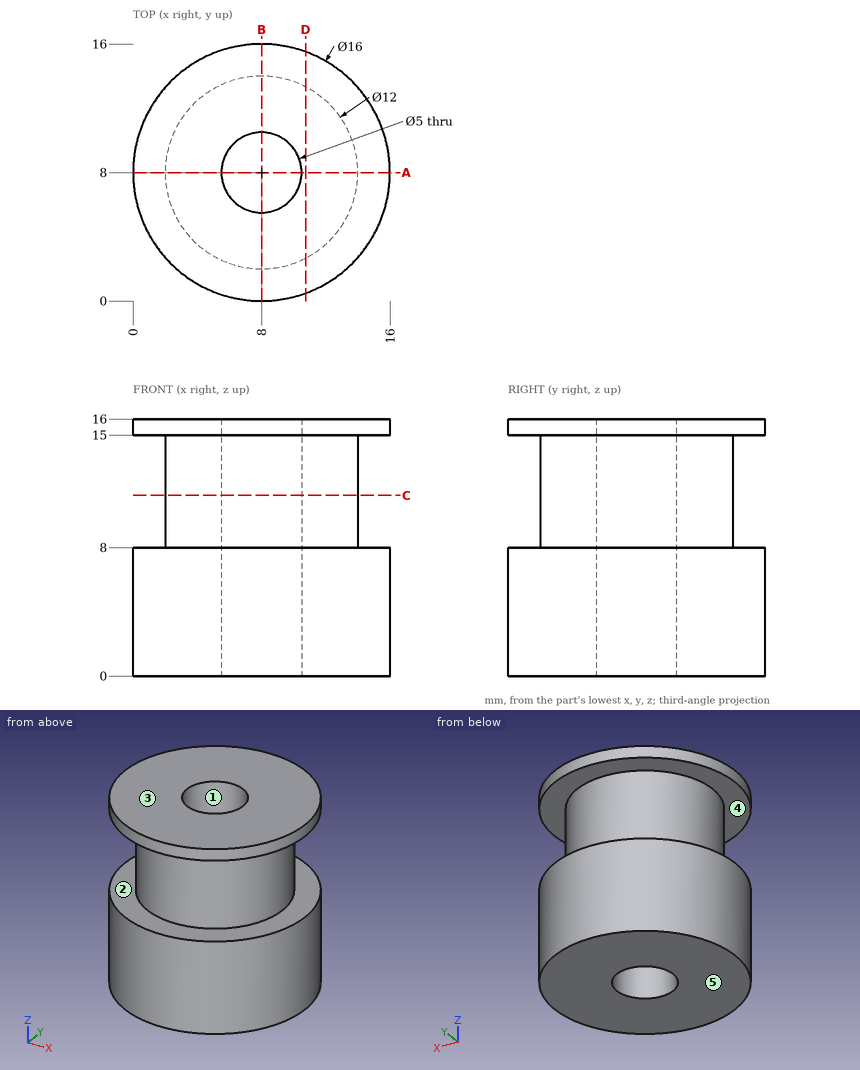
Part print with two shaded views. Sizes in mm from the minimum x, y, z corner. A direction names the side the tool comes from. Round coordinates to 2 decimals unless told otherwise and drop trailing zeros. Order: outer loops, then holes, each group sorted by start corner. A loop starts at its lowest first (then second) coordinate and runs counter-clockwise, first axis right, second up. Notation, with made-up numbers: (73.5, 15) -> (122.5, 15) arc R21 cw to (122.5, 51) -> close; hole circle Ø4 at (-18, 58.25). An arc over 180 degrees is marked (long way). Write each question's results on one line, items separated by ' | '.
1. Cut at C-C (z = 11.25). Give the cut face in (x, y), plus the area to 3 significant figures.
Findings below:
outline: circle Ø12 at (8, 8); hole circle Ø5 at (8, 8) | area: 93.5 mm²
2. Pull direction Z, two halves, no side cores. Call the marked faces 3, 4 and 5: pulls with the +Z half, pulls with the -Z half, needs draft (parallel to the pull), parting line crosses it, or undercut.
Findings below:
face 3: pulls with the +Z half | face 4: undercut | face 5: pulls with the -Z half
3. Cut at D-D (x = 10.75). Give the cut face in (y, z), plus the area to 3 significant figures.
Findings below:
outline: (0.49, 0) -> (15.51, 0) -> (15.51, 8) -> (13.33, 8) -> (13.33, 15) -> (15.51, 15) -> (15.51, 16) -> (0.49, 16) -> (0.49, 15) -> (2.67, 15) -> (2.67, 8) -> (0.49, 8) -> close | area: 210 mm²
4. Cut at A-A (y = 8). Give the cut face in (x, z), plus the area to 3 significant figures.
Findings below:
outline: (0, 0) -> (5.5, 0) -> (5.5, 16) -> (0, 16) -> (0, 15) -> (2, 15) -> (2, 8) -> (0, 8) -> close; (10.5, 0) -> (16, 0) -> (16, 8) -> (14, 8) -> (14, 15) -> (16, 15) -> (16, 16) -> (10.5, 16) -> close | area: 148 mm²
5. 3-axis set-ups, long thin cutter, end or side, ignore diameter. For the marked faces 1 and 2: which of +Z, -Z, +X, -X, +Y, -Y reach the whole face in a straight line?
Findings below:
face 1: +Z, -Z | face 2: none
6. Wall check: line 1 along Y through (x, z) = (8, 5.5); line 2 along Y through (x, z) = (8, 9); line 3 along Z through (x, y) = (2, 12.5). Give the ranges that are in metal, low to high. Write a range as [from, to].
Findings below:
line 1: y = [0, 5.5], [10.5, 16] | line 2: y = [2, 5.5], [10.5, 14] | line 3: z = [0, 8], [15, 16]
7. Flat gauge pins, fed straight in: P1, Ø3, axis at y = 5.5, z = 14, coming from the -X side; P2, Ø2, axis at y = 2.5, z = 10.5, coming from the -X side; P3, Ø8, axis at x = 4, z = 13, coming from the +Y side. Where does each tip first touch, or does it go through?
Findings below:
P1: stops at x = 0.12 | P2: stops at x = 4.03 | P3: stops at y = 15.98
